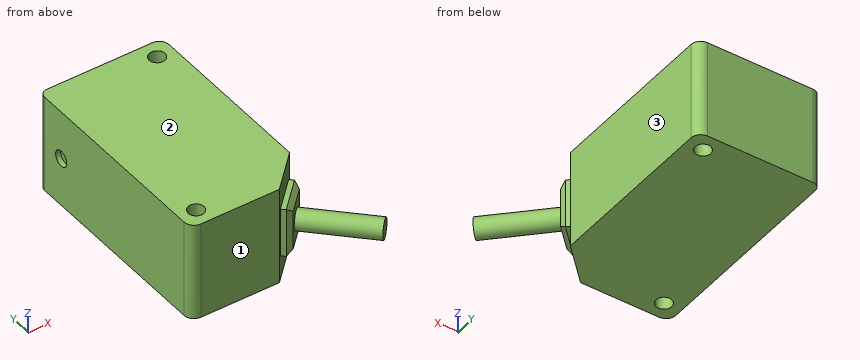
from build123d import *

# Parameters (mm, degrees)
SKETCH_1_R          = 1.6
EXTRUDE_1_DEPTH     = 20
SKETCH_2_R          = 1.6
CUT_EXTRUDE_1_DEPTH = 1
FILLET_1_R          = 1.5
FILLET_2_R          = 2
SKETCH_3_W          = 10
SKETCH_3_H          = 8
EXTRUDE_2_DEPTH     = 2
CHAMFER_1_SIZE      = 1
SKETCH_4_R          = 2
EXTRUDE_3_DEPTH     = 15


with BuildPart() as part:
    # 草图1 → 凸台-拉伸1 (new body)
    with BuildSketch(Plane.XY):
        Polygon((0, 0), (0, 44), (25, 44), (25, 7), (18, 0), align=None)
        with Locations((21.5, 40.5)):
            Circle(SKETCH_1_R, mode=Mode.SUBTRACT)
        with Locations((3.5, 3.5)):
            Circle(SKETCH_1_R, mode=Mode.SUBTRACT)
    extrude(amount=EXTRUDE_1_DEPTH)

    # 草图2 → 切除-拉伸1 (cut)
    with BuildSketch(Plane.ZY):
        with Locations(Location((10, 37.7, 0), (0, 0, 270))):
            Circle(SKETCH_2_R)
    extrude(amount=-CUT_EXTRUDE_1_DEPTH, mode=Mode.SUBTRACT)

    # 圆角1
    fillet_1_edges = [part.edges().sort_by_distance(p)[0] for p in [
        (0, 44, 10),
    ]]
    fillet(fillet_1_edges, radius=FILLET_1_R)

    # 圆角2
    fillet_2_edges = [part.edges().sort_by_distance(p)[0] for p in [
        (0, 0, 10),
        (25, 44, 10),
    ]]
    fillet(fillet_2_edges, radius=FILLET_2_R)

    # 草图3 → 凸台-拉伸2 (add)
    with BuildSketch(Plane(origin=(9, -9, 0), x_dir=(0, 0, -1), z_dir=(0.7071067811865487, -0.7071067811865464, 0))):
        with Locations((-10, 17.67766953)):
            Rectangle(SKETCH_3_W, SKETCH_3_H)
    extrude(amount=EXTRUDE_2_DEPTH)

    # 倒角1
    chamfer_1_edges = [part.edges().sort_by_distance(p)[0] for p in [
        (22.914213562, 2.085786438, 5),
        (25.742640687, 4.914213562, 10),
        (22.914213562, 2.085786438, 15),
        (20.085786438, -0.742640687, 10),
    ]]
    chamfer(chamfer_1_edges, length=CHAMFER_1_SIZE)

    # 草图4 → 凸台-拉伸3 (add)
    with BuildSketch(Plane(origin=(10.414213562, -10.414213562, 0), x_dir=(0, 0, -1), z_dir=(0.7071067811865485, -0.7071067811865467, 0))):
        with Locations(Location((-10, 17.67766953, 0), (0, 0, 90))):
            Circle(SKETCH_4_R)
    extrude(amount=EXTRUDE_3_DEPTH)


solid = part.part
Source: CAD feature listing. Evaluate the final solid. Frame: model axes, mm. Face numbers are marked on the shaded views. A direction names the side the tool comes from. Round coordinates to 2 decimals unless told otherwise and drop trailing zeros. Order: outer loops, then holes, each group sorted by start corner. A loop starts at its lowest first (then second) coordinate and runs counter-clockwise, first axis right, second up. Notation, with made-up numbers: (79, -9) - (100, -9) arc R21 cw to (100, 5) - close; hole circle Ø4 at (-36.5, 35.25). An arc over 180 degrees is marked (long way). Use a Markdown table: item, result. Add a question column.
1. Section query A-A (z = 10). Return the cut outline in (x, y).
2. Section query B-B (x = 3.5). Return the cut outline in (y, z), then the cut area to 3 significant figures.
3. Section query D-D (z = 17.25). Return the cut outline in (x, y).
4. Section query C-C (y = 37.7). Return the cut outline in (x, z), then the cut area to 3 significant figures.
5. Line query: probe 1 along Z at (x, y) = (0.6, 37.7); probe 2 along X at (y, z) = (32, 8.25); probe 3 along Y at (x, z) = (13, 9). Output: solid intervals per line, ascending.
6. Set-up query: the marked faces 1, 2 and 3. Return all of +Z, -Z, +X, -X, +Y, -Y with unobstructed straight access to the full face (end or side cutting, diameter ignored); none if empty.
7. First-contact query: pin 1 (1 mm diameter, centred on y = 38.5, z = 10.5, fed in from -X); pin 2 (0.7 mm diameter, centred on x = 20, z = 11, fed in from -Y); pin 3 (10 mm diameter, centred on x = 29.5, z = 5.5, fed in from -Y). Flat tips, straight axial feed; report the tip coordinate or a pass-through.
Derived:
| question | item | result |
|---|---|---|
| 1 | outline | (0, 2) arc R2 ccw to (2, 0) - (18, 0) - (18.67, 0.67) - (19.38, -0.04) - (20.79, -0.04) - (21.5, 0.67) - (32.11, -9.94) - (34.94, -7.11) - (24.33, 3.5) - (25.04, 4.21) - (25.04, 5.62) - (24.33, 6.33) - (25, 7) - (25, 42) arc R2 ccw to (23, 44) - (1.5, 44) arc R1.5 ccw to (0, 42.5) - (0, 39.3) - (1, 39.3) - (1, 36.1) - (0, 36.1) - close; hole circle Ø3.2 at (3.5, 3.5); hole circle Ø3.2 at (21.5, 40.5) |
| 2 | outline | (0, 0) - (1.9, 0) - (1.9, 20) - (0, 20) - close; (5.1, 0) - (44, 0) - (44, 20) - (5.1, 20) - close |
| 2 | area | 816 mm2 |
| 3 | outline | (0, 2) arc R2 ccw to (2, 0) - (18, 0) - (25, 7) - (25, 42) arc R2 ccw to (23, 44) - (1.5, 44) arc R1.5 ccw to (0, 42.5) - close; hole circle Ø3.2 at (3.5, 3.5); hole circle Ø3.2 at (21.5, 40.5) |
| 4 | outline | (0, 0) - (25, 0) - (25, 20) - (0, 20) - (0, 11.6) - (1, 11.6) - (1, 8.4) - (0, 8.4) - close |
| 4 | area | 497 mm2 |
| 5 | probe 1 | 0 to 8.4, 11.6 to 20 |
| 5 | probe 2 | 0 to 25 |
| 5 | probe 3 | 0 to 44 |
| 6 | face 1 | +Z, -Z, -X, -Y |
| 6 | face 2 | +Z, +X, -X, +Y, -Y |
| 6 | face 3 | +Z, -Z, +X, +Y |
| 7 | pin 1 | x = 1 |
| 7 | pin 2 | y = -0.04 |
| 7 | pin 3 | y = -9.92 |
